Check sheet for the modelled part. Datum: model origin and axes. Units: mm. Face numbers are marked on the shaded views. A direction names the side the tool comes from. Round coordinates to 2 decimals unless told otherwise and drop trailing zeros. Order: outer loops, then holes, each group sorted by start corner. A loop starts at its lowest first (then second) coordinate and runs counter-clockwise, first axis right, second up.
(1) Tool access check on the marked faces 4, 5, 6 and 7. Record the directions out of +Z, -Z, +X, -X, +Y, -Y that give a thin tool (end or side, any length) a straight path to the whole face; none if there is none.
(2) Thickness scan on probe 1 along Z at (x, y) = (33, 30) (3 decimals); probe 2 along X at (y, z) = (-23, 28); probe 3 along X at (y, z) = (-49, -0.5) (3 decimals). Record the ranges inside material, lowest first.
(3) Mould release check, pull along X, two halves, no side actions. Record for the marked faces 1, 2 and 3: released by +X, released by -X, zero draft, split by the parting line, or undercut.
(4) Sectioned sample at B-B, the plane y = -51.5. Enter the section's corners in (x, z) (3 decimals), and give its area (3 significant figures).
(5) Sectioned sample at A-A, the plane z = -4. Enter the section's corners in (x, y) (3 decimals), and give its area (3 significant figures).
(6) Sectioned sample at C-C, the plane x = 96.5. Enter the section's corners in (y, z) (3 decimals).
(7) Depth check by flat-ended pin: pin 1 (15 mm diameter, centred on x = 85, y = 2, fed in from -Z); pin 2 (3 mm diameter, centred on x = 38, z = 22, fed in from +Y); pin 3 (15.5 mm diameter, centred on x = 7, z = 46, fed in from +Y). Enter the tip coordinate at first touch or a pass-through.
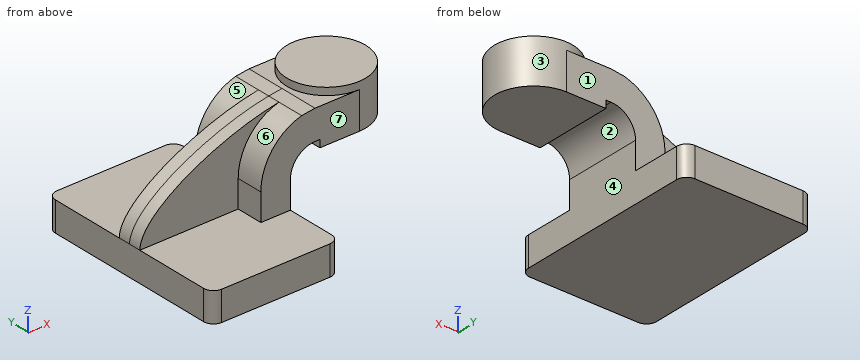
```python
from build123d import *

# Parameters (mm, degrees)
F1_DEPTH = 63.5
F2_DEPTH = 25.4
F3_DEPTH = 7.9375
F5_R     = 6.35


with BuildPart() as f1:
    # F0 (on Front) → F1 (new body, symmetric)
    with BuildSketch(Plane.XZ):
        Polygon((22.225, 9.525), (-41.275, 9.525), (-41.275, -9.525), (41.275, -9.525), (41.275, 9.525), align=None)
    extrude(amount=F1_DEPTH, both=True)

    # F0 (on Front) → F2 (join, symmetric)
    with BuildSketch(Plane.XZ):
        with BuildLine():
            Line((22.225, 27.0002), (22.225, 9.525))
            Line((22.225, 9.525), (41.275, 9.525))
            Line((41.275, 9.525), (41.275, 27.0002))
            ThreePointArc((41.275, 27.0002), (45.92468, 38.22552), (57.15, 42.8752))
            Line((57.15, 42.8752), (60.325, 42.8752))
            Line((60.325, 42.8752), (60.325, 61.9252))
            Line((60.325, 61.9252), (57.15, 61.9252))
            add(Edge.make_bspline(
                [(48.54343, 60.848133), (51.47075, 61.31001), (54.347268, 61.6721), (57.15, 61.9252)],
                knots=[103.89725, 103.89725, 103.89725, 103.89725, 111.504536, 111.504536, 111.504536, 111.504536], degree=3))
            ThreePointArc((48.54343, 60.848133), (29.578819, 48.438147), (22.225, 27.0002))
        make_face()
        Polygon((85.725, 61.9252), (60.325, 61.9252), (60.325, 42.8752), (60.325, 38.1), (85.725, 38.1), align=None)
    extrude(amount=F2_DEPTH, both=True)

    # F0 (on Front) → F3 (join, symmetric)
    with BuildSketch(Plane.XZ):
        with BuildLine():
            add(Edge.make_bspline(
                [(-41.275, 9.525), (-40.893038, 29.61845), (8.563274, 54.539999), (48.54343, 60.848133)],
                knots=[0, 0, 0, 0, 103.89725, 103.89725, 103.89725, 103.89725], degree=3))
            Line((-41.275, 9.525), (22.225, 9.525))
            Line((22.225, 9.525), (22.225, 27.0002))
            ThreePointArc((22.225, 27.0002), (29.578819, 48.438147), (48.54343, 60.848133))
        make_face()
    extrude(amount=F3_DEPTH, both=True)

    # F0 (on Front) → F4 (revolve)
    with BuildSketch(Plane.XZ):
        Polygon((85.725, 66.675), (85.725, 61.9252), (85.725, 38.1), (111.125, 38.1), (111.125, 66.675), align=None)
    revolve(axis=Axis((85.725, 0, 52.3875), (0, 0, 1)))

    # F5
    f5_edges = [f1.edges().sort_by_distance(p)[0] for p in [
        (-41.275, -63.5, 0),
        (41.275, -63.5, 0),
        (41.275, 63.5, 0),
        (-41.275, 63.5, 0),
    ]]
    fillet(f5_edges, radius=F5_R)


solid = f1.part
```
Derived:
1. face 4: -Z, +X, +Y, -Y
1. face 5: +Z, -X, +Y
1. face 6: +Z, -X, -Y
1. face 7: +Z, +X, -X, -Y
2. probe 1: z = -9.525 to 9.525
2. probe 2: x = 22.24 to 41.31
2. probe 3: x = -41.275 to 41.275
3. face 1: zero draft
3. face 2: undercut
3. face 3: split by the parting line
4. outline: (-41.275, -9.525) - (41.275, -9.525) - (41.275, 9.525) - (-41.275, 9.525) - close
4. area: 1,570 mm2
5. outline: (-41.275, -57.15) arc R6.35 ccw to (-34.925, -63.5) - (34.925, -63.5) arc R6.35 ccw to (41.275, -57.15) - (41.275, 57.15) arc R6.35 ccw to (34.925, 63.5) - (-34.925, 63.5) arc R6.35 ccw to (-41.275, 57.15) - close
5. area: 10,400 mm2
6. outline: (-23.001, 38.1) - (23.001, 38.1) - (23.001, 66.675) - (-23.001, 66.675) - close
7. pin 1: stops at z = 38.1
7. pin 2: stops at y = 25.4
7. pin 3: stops at y = 7.94
